The listing builds one solid part. Answer for the finished solid, in the listing's coordinates (mm). A direction names the side the tool comes from. Coordinates: 2 decimals unless noted, no trailing zeros. Write each loop counter-clockwise with the first axis right and the second up, starting at its lowest first coordinate (ties: lowest second). Pieces come first, ordered by that corner, then holes.
from build123d import *

# Parameters (mm, degrees)
SKETCH_1_R          = 70
EXTRUDE_1_DEPTH     = 35
EXTRUDE_2_DEPTH     = 3.5
CHAMFER_1_SIZE      = 1
SKETCH_3_R          = 40
CUT_EXTRUDE_1_DEPTH = 6
SKETCH_5_R          = 4.6
CUT_EXTRUDE_2_DEPTH = 49
SKETCH_6_R          = 70
SKETCH_6_R_2        = 55
CUT_EXTRUDE_3_DEPTH = 6
SKETCH_7_R          = 6.75
CUT_EXTRUDE_4_DEPTH = 8.5
SKETCH_8_R          = 4
CUT_EXTRUDE_5_DEPTH = 40.5
SKETCH_9_R          = 22.5
CUT_EXTRUDE_6_DEPTH = 49.5


with BuildPart() as part:
    # 草图1 → 凸台-拉伸1 (new body)
    with BuildSketch(Plane.XY):
        Circle(SKETCH_1_R)
    extrude(amount=EXTRUDE_1_DEPTH)

    # 草图2 → 凸台-拉伸2 (add)
    with BuildSketch(Plane.XY.offset(35)):
        with BuildLine():
            Line((60, 0), (70, 0))
            ThreePointArc((70, 0), (69.489621187, 8.437567618), (67.96592722, 16.7520965))
            Line((67.96592722, 16.7520965), (58.256509046, 14.358939857))
            ThreePointArc((58.256509046, 14.358939857), (59.562532446, 7.232200815), (60, 0))
        make_face()
        with BuildLine():
            Line((53.127361539, 27.883390323), (61.981921796, 32.530622043))
            ThreePointArc((61.981921796, 32.530622043), (57.608870613, 39.764532271), (52.395752372, 46.418586077))
            Line((52.395752372, 46.418586077), (44.91064489, 39.787359494))
            ThreePointArc((44.91064489, 39.787359494), (49.379031954, 34.083884804), (53.127361539, 27.883390323))
        make_face()
        with BuildLine():
            Line((34.083884804, 49.379031954), (39.764532271, 57.608870613))
            ThreePointArc((39.764532271, 57.608870613), (32.530622043, 61.981921796), (24.822342093, 65.451136988))
            Line((24.822342093, 65.451136988), (21.276293223, 56.100974561))
            ThreePointArc((21.276293223, 56.100974561), (27.883390323, 53.127361539), (34.083884804, 49.379031954))
        make_face()
        with BuildLine():
            Line((7.232200815, 59.562532446), (8.437567618, 69.489621187))
            ThreePointArc((8.437567618, 69.489621187), (0, 70), (-8.437567618, 69.489621187))
            Line((-8.437567618, 69.489621187), (-7.232200815, 59.562532446))
            ThreePointArc((-7.232200815, 59.562532446), (0, 60), (7.232200815, 59.562532446))
        make_face()
        with BuildLine():
            Line((-21.276293223, 56.100974561), (-24.822342093, 65.451136988))
            ThreePointArc((-24.822342093, 65.451136988), (-32.530622043, 61.981921796), (-39.764532271, 57.608870613))
            Line((-39.764532271, 57.608870613), (-34.083884804, 49.379031954))
            ThreePointArc((-34.083884804, 49.379031954), (-27.883390323, 53.127361539), (-21.276293223, 56.100974561))
        make_face()
        with BuildLine():
            Line((-44.91064489, 39.787359494), (-52.395752372, 46.418586077))
            ThreePointArc((-52.395752372, 46.418586077), (-57.608870613, 39.764532271), (-61.981921796, 32.530622043))
            Line((-61.981921796, 32.530622043), (-53.127361539, 27.883390323))
            ThreePointArc((-53.127361539, 27.883390323), (-49.379031954, 34.083884804), (-44.91064489, 39.787359494))
        make_face()
        with BuildLine():
            Line((-58.256509046, 14.358939857), (-67.96592722, 16.7520965))
            ThreePointArc((-67.96592722, 16.7520965), (-69.489621187, 8.437567618), (-70, 0))
            Line((-70, 0), (-60, 0))
            ThreePointArc((-60, 0), (-59.562532446, 7.232200815), (-58.256509046, 14.358939857))
        make_face()
        with BuildLine():
            Line((-58.256509046, -14.358939857), (-67.96592722, -16.7520965))
            ThreePointArc((-67.96592722, -16.7520965), (-65.451136988, -24.822342093), (-61.981921796, -32.530622043))
            Line((-61.981921796, -32.530622043), (-53.127361539, -27.883390323))
            ThreePointArc((-53.127361539, -27.883390323), (-56.100974561, -21.276293223), (-58.256509046, -14.358939857))
        make_face()
        with BuildLine():
            Line((-44.91064489, -39.787359494), (-52.395752372, -46.418586077))
            ThreePointArc((-52.395752372, -46.418586077), (-46.418586077, -52.395752372), (-39.764532271, -57.608870613))
            Line((-39.764532271, -57.608870613), (-34.083884804, -49.379031954))
            ThreePointArc((-34.083884804, -49.379031954), (-39.787359494, -44.91064489), (-44.91064489, -39.787359494))
        make_face()
        with BuildLine():
            Line((-21.276293223, -56.100974561), (-24.822342093, -65.451136988))
            ThreePointArc((-24.822342093, -65.451136988), (-16.7520965, -67.96592722), (-8.437567618, -69.489621187))
            Line((-8.437567618, -69.489621187), (-7.232200815, -59.562532446))
            ThreePointArc((-7.232200815, -59.562532446), (-14.358939857, -58.256509046), (-21.276293223, -56.100974561))
        make_face()
        with BuildLine():
            Line((7.232200815, -59.562532446), (8.437567618, -69.489621187))
            ThreePointArc((8.437567618, -69.489621187), (16.7520965, -67.96592722), (24.822342093, -65.451136988))
            Line((24.822342093, -65.451136988), (21.276293223, -56.100974561))
            ThreePointArc((21.276293223, -56.100974561), (14.358939857, -58.256509046), (7.232200815, -59.562532446))
        make_face()
        with BuildLine():
            Line((34.083884804, -49.379031954), (39.764532271, -57.608870613))
            ThreePointArc((39.764532271, -57.608870613), (46.418586077, -52.395752372), (52.395752372, -46.418586077))
            Line((52.395752372, -46.418586077), (44.91064489, -39.787359494))
            ThreePointArc((44.91064489, -39.787359494), (39.787359494, -44.91064489), (34.083884804, -49.379031954))
        make_face()
        with BuildLine():
            Line((53.127361539, -27.883390323), (61.981921796, -32.530622043))
            ThreePointArc((61.981921796, -32.530622043), (65.451136988, -24.822342093), (67.96592722, -16.7520965))
            Line((67.96592722, -16.7520965), (58.256509046, -14.358939857))
            ThreePointArc((58.256509046, -14.358939857), (56.100974561, -21.276293223), (53.127361539, -27.883390323))
        make_face()
    extrude(amount=EXTRUDE_2_DEPTH)

    # 倒角1
    chamfer_1_edges = [part.edges().sort_by_distance(p)[0] for p in [
        (63.111218133, 15.555518179, 38.5),
        (69.489621187, 8.437567618, 38.5),
        (65, 0, 38.5),
        (59.562532446, 7.232200815, 38.5),
        (63.111218133, -15.555518179, 38.5),
        (65.451136988, -24.822342093, 38.5),
        (57.554641667, -30.207006183, 38.5),
        (56.100974561, -21.276293223, 38.5),
        (48.653198631, -43.102972786, 38.5),
        (46.418586077, -52.395752372, 38.5),
        (36.924208538, -53.493951283, 38.5),
        (39.787359494, -44.91064489, 38.5),
        (23.049317658, -60.776055775, 38.5),
        (16.7520965, -67.96592722, 38.5),
        (7.834884217, -64.526076816, 38.5),
        (14.358939857, -58.256509046, 38.5),
        (-7.834884217, -64.526076816, 38.5),
        (-16.7520965, -67.96592722, 38.5),
        (-23.049317658, -60.776055775, 38.5),
        (-14.358939857, -58.256509046, 38.5),
        (-36.924208538, -53.493951283, 38.5),
        (-46.418586077, -52.395752372, 38.5),
        (-48.653198631, -43.102972786, 38.5),
        (-39.787359494, -44.91064489, 38.5),
        (-57.554641667, -30.207006183, 38.5),
        (-65.451136988, -24.822342093, 38.5),
        (-63.111218133, -15.555518179, 38.5),
        (-56.100974561, -21.276293223, 38.5),
        (-65, 0, 38.5),
        (-69.489621187, 8.437567618, 38.5),
        (-63.111218133, 15.555518179, 38.5),
        (-59.562532446, 7.232200815, 38.5),
        (-48.653198631, 43.102972786, 38.5),
        (-49.379031954, 34.083884804, 38.5),
        (-57.554641667, 30.207006183, 38.5),
        (-57.608870613, 39.764532271, 38.5),
        (-23.049317658, 60.776055775, 38.5),
        (-27.883390323, 53.127361539, 38.5),
        (-36.924208538, 53.493951283, 38.5),
        (-32.530622043, 61.981921796, 38.5),
        (7.834884217, 64.526076816, 38.5),
        (0, 60, 38.5),
        (-7.834884217, 64.526076816, 38.5),
        (0, 70, 38.5),
        (36.924208538, 53.493951283, 38.5),
        (27.883390323, 53.127361539, 38.5),
        (23.049317658, 60.776055775, 38.5),
        (32.530622043, 61.981921796, 38.5),
        (57.554641667, 30.207006183, 38.5),
        (49.379031954, 34.083884804, 38.5),
        (48.653198631, 43.102972786, 38.5),
        (57.608870613, 39.764532271, 38.5),
    ]]
    chamfer(chamfer_1_edges, length=CHAMFER_1_SIZE)

    # 草图3 → 切除-拉伸1 (cut)
    with BuildSketch(Plane.XY.offset(35)):
        Circle(SKETCH_3_R)
    extrude(amount=-CUT_EXTRUDE_1_DEPTH, mode=Mode.SUBTRACT)

    # 草图5 → 切除-拉伸2 (cut)
    with BuildSketch(Plane(origin=(0, 0, 0), x_dir=(-1, 0, 0), z_dir=(0, 0, -1))):
        with Locations((-40.703193978, 23.5)):
            Circle(SKETCH_5_R)
        with Locations((40.703193978, 23.5)):
            Circle(SKETCH_5_R)
        with Locations((0, -47)):
            Circle(SKETCH_5_R)
    extrude(amount=-CUT_EXTRUDE_2_DEPTH, mode=Mode.SUBTRACT)

    # 草图6 → 切除-拉伸3 (cut)
    with BuildSketch(Plane(origin=(0, 0, 0), x_dir=(-1, 0, 0), z_dir=(0, 0, -1))):
        Circle(SKETCH_6_R)
        Circle(SKETCH_6_R_2, mode=Mode.SUBTRACT)
    extrude(amount=-CUT_EXTRUDE_3_DEPTH, mode=Mode.SUBTRACT)

    # 草图7 → 切除-拉伸4 (cut)
    with BuildSketch(Plane.XY.offset(35)):
        with Locations((51.024999685, -35.220014297)):
            Circle(SKETCH_7_R)
        with Locations((-51.024999685, -35.220014297)):
            Circle(SKETCH_7_R)
        with Locations((-41.113604811, 46.407666387)):
            Circle(SKETCH_7_R)
        with Locations((41.113604811, 46.407666387)):
            Circle(SKETCH_7_R)
    extrude(amount=-CUT_EXTRUDE_4_DEPTH, mode=Mode.SUBTRACT)

    # 草图8 → 切除-拉伸5 (cut)
    with BuildSketch(Plane.XY.offset(26.5)):
        with Locations((41.113604811, 46.407666387)):
            Circle(SKETCH_8_R)
        with Locations((51.024999685, -35.220014297)):
            Circle(SKETCH_8_R)
        with Locations((-51.024999685, -35.220014297)):
            Circle(SKETCH_8_R)
        with Locations((-41.113604811, 46.407666387)):
            Circle(SKETCH_8_R)
    extrude(amount=-CUT_EXTRUDE_5_DEPTH, mode=Mode.SUBTRACT)

    # 草图9 → 切除-拉伸6 (cut)
    with BuildSketch(Plane.XY.offset(29)):
        Circle(SKETCH_9_R)
    extrude(amount=-CUT_EXTRUDE_6_DEPTH, mode=Mode.SUBTRACT)


solid = part.part
1. For a pull along X with two mould halves and no side action, classify faces 1 (the flat face through (63.058, -16.065, 38.007)), 2 (the conical face through (-28.158, 53.43, 37.896)), 3 (the conical face through (-57.03, 39.51, 38.12)) as pulls with the +X half, pulls with the -X half, needs draft (parallel to the pull), parting line crosses it, or undercut.
Results found:
face 1: pulls with the +X half
face 2: undercut
face 3: pulls with the -X half
2. Find the intervals of material crossed by L1, parallel to Y at x = 0, z = 23.5; L2, parallel to Y at x = -41, z = 13.5; L3, parallel to X at y = 23, z = 25, in increasing order.
Results found:
L1: y = -70 to -51.6, -42.4 to -22.5, 22.5 to 70
L2: y = -56.74 to 18.91, 28.09 to 42.41, 50.41 to 56.74
L3: x = -66.11 to -45.28, -36.13 to 36.13, 45.28 to 66.11
3. Section D-D on z = 21.5 is taken. State how many separate pieces and enclosed holes the cut face has, then the cut area to 3 significant figures.
Results found:
separate pieces: 1
enclosed holes: 8
area: 13,400 mm2
4. Flat-ended cylindrical pins translate along their axes: P1, Ø5, axis at y = -30.5, z = 22.5, coming from the -X side; P2, Ø6, axis at y = 7.5, z = 9, coming from the -X side; P3, Ø15, axis at x = -40, y = 44, coming from the +Z side. Find the tip coordinate at first contact, or state that the pin passes through.
Results found:
P1: stops at x = -64.16
P2: stops at x = -69.86
P3: stops at z = 38.38
5. Section A-A on x = 0 is taken. Give the vertices of the cut face in (y, z).
Results found:
outline: (-70, 6) - (-55, 6) - (-55, 0) - (-51.6, 0) - (-51.6, 35) - (-70, 35) - close; (-42.4, 0) - (-22.5, 0) - (-22.5, 29) - (-40, 29) - (-40, 35) - (-42.4, 35) - close; (22.5, 0) - (55, 0) - (55, 6) - (70, 6) - (70, 37.5) - (69, 38.5) - (61, 38.5) - (60, 37.5) - (60, 35) - (40, 35) - (40, 29) - (22.5, 29) - close
6. Section C-C on y = -5.5 is taken. Give the vertices of the cut face in (x, z), then the cut area to 3 significant figures.
Results found:
outline: (-69.78, 6) - (-54.72, 6) - (-54.72, 0) - (-21.82, 0) - (-21.82, 29) - (-39.62, 29) - (-39.62, 35) - (-69.78, 35) - close; (21.82, 0) - (54.72, 0) - (54.72, 6) - (69.78, 6) - (69.78, 35) - (39.62, 35) - (39.62, 29) - (21.82, 29) - close
area: 2,960 mm2
7. Section B-B on z = 4 is taken. Give the vertices of the cut face in (x, y), then the cut area to 3 significant figures.
Results found:
outline: circle Ø110 at (0, 0); hole circle Ø9.2 at (-40.7, 23.5); hole circle Ø45 at (0, 0); hole circle Ø9.2 at (0, -47); hole circle Ø9.2 at (40.7, 23.5)
area: 7,710 mm2
8. A tool of negligible diameter and unlimited length cuts with its end or side. For faces 4 (the flat face through (-23.5, 60.53, 38.01)), 5 (the cylindrical face through (27.793, 53.174, 36.232)), 6 (the conical face through (64.83, -24.71, 38.12)), from which of +Z, -Z, +X, -X, +Y, -Y can it reach the whole face along a straight path? Write none if from no direction.
Results found:
face 4: +Z, +Y
face 5: +Z
face 6: +Z, +X, -Y
